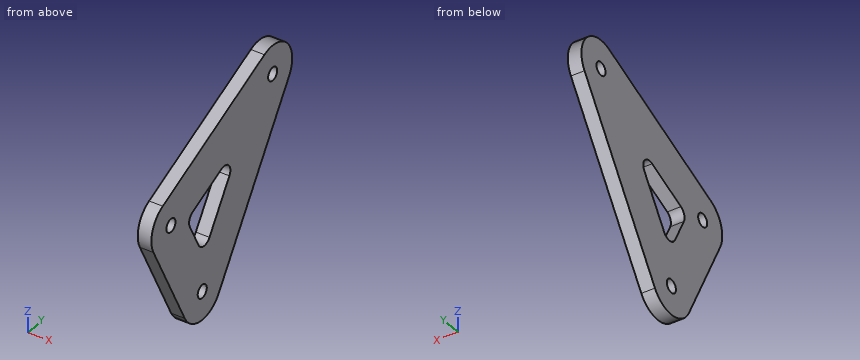
```python
from build123d import *

# Parameters (mm, degrees)
SKETCH1_R           = 6.25
SKETCH1_R_2         = 1.45
BOSS_EXTRUDE1_DEPTH = 1.5
CUT_EXTRUDE1_DEPTH  = 3


with BuildPart() as part:
    # Sketch1 → Boss-Extrude1 (new body, symmetric)
    with BuildSketch(Plane(origin=(0, 0, 0), x_dir=(0, 0, -1), z_dir=(1, 0, 0))):
        with Locations((20, 10.000000011)):
            Circle(SKETCH1_R)
        with Locations((20, 10.000000011)):
            Circle(SKETCH1_R_2, mode=Mode.SUBTRACT)
        with BuildLine():
            ThreePointArc((-8.75, 32.5), (-13.659228479, 26.395507251), (-20.674746153, 29.880886391))
            Line((-20.674746153, 29.880886391), (-5.674746153, -2.619113609))
            ThreePointArc((-5.674746153, -2.619113609), (-1.340771521, 6.104492749), (6.25, 0))
            ThreePointArc((6.25, 0), (5.316567553, -3.28581945), (2.795084974, -5.590169942))
            Line((2.795084974, -5.590169942), (22.795084974, 4.409830069))
            ThreePointArc((22.795084974, 4.409830069), (13.759058052, 10.336368263), (23.379734945, 15.257365483))
            Line((23.379734945, 15.257365483), (-11.620265055, 37.757365472))
            ThreePointArc((-11.620265055, 37.757365472), (-9.514298431, 35.494925425), (-8.75, 32.5))
        make_face()
        Circle(SKETCH1_R)
        Circle(SKETCH1_R_2, mode=Mode.SUBTRACT)
        with Locations((-15, 32.5)):
            Circle(SKETCH1_R)
        with Locations((-15, 32.5)):
            Circle(SKETCH1_R_2, mode=Mode.SUBTRACT)
    extrude(amount=BOSS_EXTRUDE1_DEPTH, both=True)

    # Sketch2 → Cut-Extrude1 (cut)
    with BuildSketch(Plane(origin=(1.5, 0, 0), x_dir=(0, 0, -1), z_dir=(1, 0, 0))):
        with BuildLine():
            Line((3.629133347, 6.007194134), (9.288126649, 8.836690789))
            ThreePointArc((9.288126649, 8.836690789), (10.390800881, 10.51790733), (9.47521464, 12.307902121))
            Line((9.47521464, 12.307902121), (-0.428023639, 18.674269583))
            ThreePointArc((-0.428023639, 18.674269583), (-2.822182558, 18.500874667), (-3.32545759, 16.153796277))
            Line((-3.32545759, 16.153796277), (0.918787386, 6.957932161))
            ThreePointArc((0.918787386, 6.957932161), (2.072692273, 5.908791877), (3.629133347, 6.007194134))
        make_face()
    extrude(amount=-CUT_EXTRUDE1_DEPTH, mode=Mode.SUBTRACT)


solid = part.part
```
Source: CAD feature listing. Evaluate the final solid. Frame: model axes, mm. Coordinates: 2 decimals unless noted, no trailing zeros. Order: outer loops, then holes, each group sorted by start corner. A loop starts at its lowest first (then second) coordinate and runs counter-clockwise, first axis right, second up. Notation, with made-up numbers: (40.5, 70) - (71.5, 70) arc R28 ccw to (71.5, 102) - close; hole circle Ø3 at (-39.75, 89.25). An arc over 180 degrees is marked (long way). One line per item, written item: value.
1) Contact query for a flat-ended pin moving along its axis: pin 1 (2.5 mm diameter, centred on y = 0, z = 0, fed in from -X). Output: stop coordinate, or through.
Computed values:
pin 1: passes through
2) Ray query, line 1 (Y direction, x = -0.25, z = 0); line 2 (Z direction, x = 1.2, y = 9.5); line 3 (Z direction, x = 0.55, y = 12). Return the intervals inside material, ascending. Write a range as [from, to].
Computed values:
line 1: y = [-6.25, -1.45], [1.45, 8.95], [18.4, 30.29]
line 2: z = [-26.23, -21.36], [-18.64, -10.05], [0.25, 11.27]
line 3: z = [-25.92, -9.85], [1.41, 12.42]
3) Cut plane C-C on y = 0. Output: boundary loops of the cut face in (x, z).
Computed values:
outline: (-1.5, -13.98) - (1.5, -13.98) - (1.5, -1.45) - (-1.5, -1.45) - close; (-1.5, 1.45) - (1.5, 1.45) - (1.5, 6.88) - (-1.5, 6.88) - close
4) Cut plane B-B on z = -20. Output: boundary loops of the cut face in (x, y), plus the area to 3 significant figures.
Computed values:
outline: (-1.5, 3.01) - (1.5, 3.01) - (1.5, 8.55) - (-1.5, 8.55) - close; (-1.5, 11.45) - (1.5, 11.45) - (1.5, 17.43) - (-1.5, 17.43) - close
area: 34.6 mm^2
5) Cut plane A-A on x = -0.9. Output: boundary loops of the cut face in (y, z), plus the area to 3 significant figures.
Computed values:
outline: (-5.59, -2.8) - (4.41, -22.8) arc R6.25 ccw to (15.26, -23.38) - (37.76, 11.62) arc R6.25 ccw to (29.88, 20.67) - (-2.62, 5.67) arc R6.25 ccw to start; hole circle Ø2.9 at (0, 0); hole (6.01, -3.63) - (8.84, -9.29) arc R2 ccw to (12.31, -9.48) - (18.67, 0.43) arc R2 ccw to (16.15, 3.33) - (6.96, -0.92) arc R2 ccw to start; hole circle Ø2.9 at (10, -20); hole circle Ø2.9 at (32.5, 15)
area: 1,030 mm^2
6) Cut plane D-D on y = 10. Output: boundary loops of the cut face in (x, z), plus the area to 3 significant figures.
Computed values:
outline: (-1.5, -26.25) - (1.5, -26.25) - (1.5, -21.45) - (-1.5, -21.45) - close; (-1.5, -18.55) - (1.5, -18.55) - (1.5, -10.29) - (-1.5, -10.29) - close; (-1.5, 0.49) - (1.5, 0.49) - (1.5, 11.5) - (-1.5, 11.5) - close
area: 72.2 mm^2
